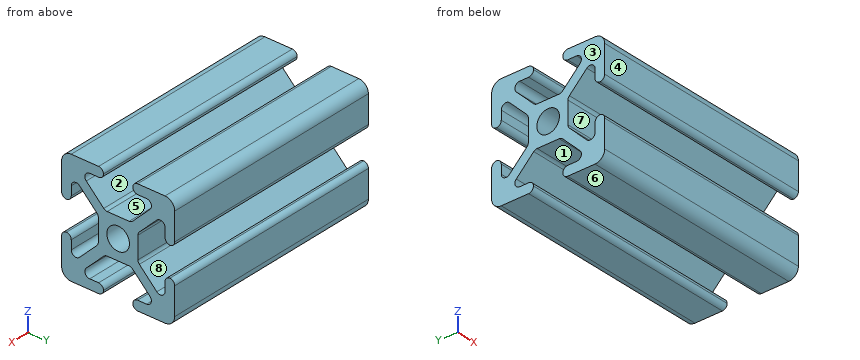
from build123d import *

# Parameters (mm, degrees)
SKETCH1_R           = 2.5
BOSS_EXTRUDE1_DEPTH = 50
FILLET1_R           = 1.065
FILLET2_R           = 2.13


with BuildPart() as part:
    # Sketch1 → Boss-Extrude1 (new body)
    with BuildSketch(Plane.YZ):
        Polygon((-12.5, -3.25), (-12.5, -12.5), (-3.25, -12.5), (-3.25, -10.37), (-8.863862556, -10.37), (-2.873862556, -4.38), (2.873862556, -4.38), (8.863862556, -10.37), (3.25, -10.37), (3.25, -12.5), (12.5, -12.5), (12.5, -3.25), (10.37, -3.25), (10.37, -8.863862556), (4.38, -2.873862556), (4.38, 2.873862556), (10.37, 8.863862556), (10.37, 3.25), (12.5, 3.25), (12.5, 12.5), (3.25, 12.5), (3.25, 10.37), (8.863862556, 10.37), (2.873862556, 4.38), (-2.873862556, 4.38), (-8.863862556, 10.37), (-3.25, 10.37), (-3.25, 12.5), (-12.5, 12.5), (-12.5, 3.25), (-10.37, 3.25), (-10.37, 8.863862556), (-4.38, 2.873862556), (-4.38, -2.873862556), (-10.37, -8.863862556), (-10.37, -3.25), align=None)
        with Locations(Location((0, 0, 0), (0, 0, 270))):
            Circle(SKETCH1_R, mode=Mode.SUBTRACT)
    extrude(amount=BOSS_EXTRUDE1_DEPTH)

    # Fillet1
    fillet1_edges = [part.edges().sort_by_distance(p)[0] for p in [
        (25, -10.37, -8.863862556),
        (25, 2.873862556, -4.38),
        (25, -2.873862556, -4.38),
        (25, -4.38, 2.873862556),
        (25, -4.38, -2.873862556),
        (25, -2.873862556, 4.38),
        (25, 2.873862556, 4.38),
        (25, 4.38, 2.873862556),
        (25, 4.38, -2.873862556),
        (25, -8.863862556, -10.37),
        (25, 8.863862556, -10.37),
        (25, 10.37, -8.863862556),
        (25, -10.37, 8.863862556),
        (25, -8.863862556, 10.37),
        (25, 10.37, 8.863862556),
        (25, 8.863862556, 10.37),
        (25, 12.5, 3.25),
        (25, -3.25, -12.5),
        (25, -10.37, 3.25),
        (25, 10.37, 3.25),
        (25, -10.37, -3.25),
        (25, -12.5, -3.25),
        (25, -12.5, 3.25),
        (25, 3.25, -10.37),
        (25, -3.25, -10.37),
        (25, 3.25, -12.5),
        (25, 10.37, -3.25),
        (25, 12.5, -3.25),
        (25, 3.25, 12.5),
        (25, 3.25, 10.37),
        (25, -3.25, 10.37),
        (25, -3.25, 12.5),
    ]]
    fillet(fillet1_edges, radius=FILLET1_R - 0.0001)  # a hair under: the kernel refuses the full size

    # Fillet2
    fillet2_edges = [part.edges().sort_by_distance(p)[0] for p in [
        (25, -12.5, 12.5),
        (25, 12.5, 12.5),
        (25, 12.5, -12.5),
        (25, -12.5, -12.5),
    ]]
    fillet(fillet2_edges, radius=FILLET2_R)


solid = part.part
Design review of the part built by this model. Coordinates are the model's own, in mm. Face numbers are marked on the shaded views. A direction names the side the tool comes from. Coordinates: 2 decimals unless noted, no trailing zeros. Order: outer loops, then holes, each group sorted by start corner. A loop starts at its lowest first (then second) coordinate and runs counter-clockwise, first axis right, second up. Notation, with made-up numbers: M 15.25,25 L 48.25,25 A29 ccw 48.25,46 Z; hole C 13.5,85 d5. An arc over 180 degrees is marked long. Use a Markdown table: item, result.
(1) Add section C-C (z = -5.5). Give the boundary of the cut face in (x, y).
Worked answers:
| item | result |
|---|---|
| outline | M 0,-12.5 L 50,-12.5 L 50,-10.37 L 0,-10.37 Z; M 0,-7.01 L 50,-7.01 L 50,-3.99 L 0,-3.99 Z; M 0,3.99 L 50,3.99 L 50,7.01 L 0,7.01 Z; M 0,10.37 L 50,10.37 L 50,12.5 L 0,12.5 Z |
(2) For P1, Ø1.5, axis at x = 26, z = -1, coming from the -Y side; P2, Ø4, axis at x = 35, y = -2, coming from the -Z side; P3, Ø2.5, axis at x = 18, z = 0, coming from the +Y side, all flat-tipped, find the tip position at first contact; note any pin that passes through.
Worked answers:
| item | result |
|---|---|
| P1 | stops at y = -4.38 |
| P2 | stops at z = -12.45 |
| P3 | stops at y = 4.38 |
(3) Wall thickness on probe 1 along Y at (x, z) = (26, 0); probe 2 along Y at (x, z) = (19.5, 4); probe 3 along Z at (x, y) = (40.5, -4.5): over which ranges is each line inside the solid? List them lowest first.
Worked answers:
| item | result |
|---|---|
| probe 1 | y = -4.38 to -2.5, 2.5 to 4.38 |
| probe 2 | y = -12.45 to -10.42, -5.51 to 5.51, 10.42 to 12.45 |
| probe 3 | z = -12.5 to -10.37, -6.01 to -2.92, 2.92 to 6.01, 10.37 to 12.5 |
(4) Draft analysis for pull direction Y (two halves, no side actions). For the marked faces 1, 2, 3 and 4, state which applies: released by +Y, released by -Y, zero draft, split by the parting line, or undercut.
Worked answers:
| item | result |
|---|---|
| face 1 | undercut |
| face 2 | undercut |
| face 3 | zero draft |
| face 4 | released by -Y |
(5) Add section A-A (z = 0). Give the boundary of the cut face in (x, y), then the cut area to 3 significant figures.
Worked answers:
| item | result |
|---|---|
| outline | M 0,-4.38 L 50,-4.38 L 50,-2.5 L 0,-2.5 Z; M 0,2.5 L 50,2.5 L 50,4.38 L 0,4.38 Z |
| area | 188 mm2 |
(6) For the marked faces 5, 6, 7 and 8, list the 3-axis set-ups (+Z, -Z, +X, -X, +Y, -Y) from which the entire face can be reached by the end or side of a thin tool; tool diameter is ignored.
Worked answers:
| item | result |
|---|---|
| face 5 | +Z, +X, -X |
| face 6 | -Z, +X, -X, +Y, -Y |
| face 7 | +X, -X, -Y |
| face 8 | +X, -X |
